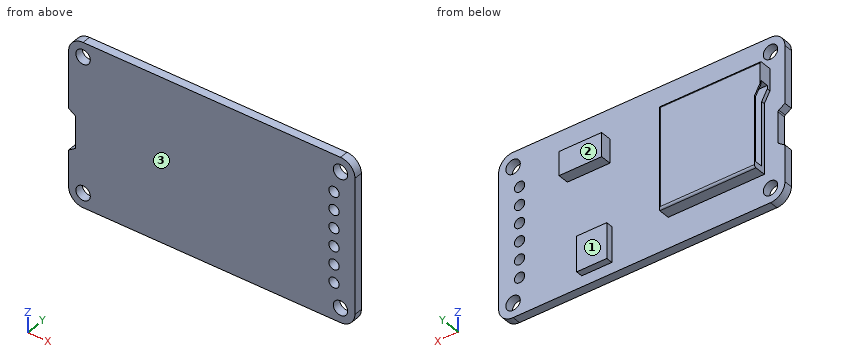
from build123d import *

# Parameters (mm, degrees)
ESQUISSE1_R                         = 1.05
PLAQUE_DEPTH                        = 1.24
CARTE_SD_DEPTH                      = 1.91
ESQUISSE4_W                         = 6.2
ESQUISSE4_H                         = 3.48
PUCE_DEPTH                          = 1.6
ESQUISSE7_W                         = 4.38
ESQUISSE7_H                         = 5.16
PUCE_2_DEPTH                        = 0.98
ESQUISSE8_R                         = 0.75
ENL_V_MAT_EXTRU_1_DEPTH             = 25.084021674
ESQUISSE9_W                         = 11.3
ESQUISSE9_H                         = 1.2
ENL_V_MAT_EXTRU_3_DEPTH             = 11.8
ENL_V_MAT_EXTRU_3_DIRECTION_2_REACH = 42.597
CONG_1_R                            = 0.3


with BuildPart() as part:
    # Esquisse1 → Plaque (new body)
    with BuildSketch(Plane(origin=(0, 0, 0), x_dir=(1, 0, 0), z_dir=(0, 1, 0))):
        with BuildLine():
            Line((-18.74, 11.92), (18.74, 11.92))
            ThreePointArc((18.74, 11.92), (20.22492424, 11.30492424), (20.84, 9.82))
            Line((20.84, 9.82), (20.84, -9.82))
            ThreePointArc((20.84, -9.82), (20.22492424, -11.30492424), (18.74, -11.92))
            Line((18.74, -11.92), (-18.74, -11.92))
            ThreePointArc((-18.74, -11.92), (-20.22492424, -11.30492424), (-20.84, -9.82))
            Line((-20.84, -9.82), (-20.84, -1.48))
            Line((-20.84, -1.48), (-19.951399946, -0.888062551))
            ThreePointArc((-19.951399946, -0.888062551), (-19.869602616, -0.798004209), (-19.84, -0.68))
            Line((-19.84, -0.68), (-19.84, 3.72))
            ThreePointArc((-19.84, 3.72), (-19.869602616, 3.838004209), (-19.951399946, 3.928062551))
            Line((-19.951399946, 3.928062551), (-20.84, 4.52))
            Line((-20.84, 4.52), (-20.84, 9.82))
            ThreePointArc((-20.84, 9.82), (-20.22492424, 11.30492424), (-18.74, 11.92))
        make_face()
        with Locations(Location((-18.74, 9.82, 0), (0, 0, 270))):
            Circle(ESQUISSE1_R, mode=Mode.SUBTRACT)
        with Locations(Location((18.74, 9.82, 0), (0, 0, 270))):
            Circle(ESQUISSE1_R, mode=Mode.SUBTRACT)
        with Locations(Location((-18.74, -9.82, 0), (0, 0, 270))):
            Circle(ESQUISSE1_R, mode=Mode.SUBTRACT)
        with Locations(Location((18.74, -9.82, 0), (0, 0, 270))):
            Circle(ESQUISSE1_R, mode=Mode.SUBTRACT)
    extrude(amount=PLAQUE_DEPTH)

    # Esquisse2 → Carte SD (add)
    with BuildSketch(Plane(origin=(0, 1.24, 0), x_dir=(1, 0, 0), z_dir=(0, 1, 0))):
        Polygon((-18.66, -7.44), (-3.84, -7.44), (-3.84, 7.44), (-17.84, 7.44), (-17.84, -2.756314418), (-18.66, -4.24), align=None)
    extrude(amount=CARTE_SD_DEPTH)

    # Esquisse4 → Puce (add)
    with BuildSketch(Plane(origin=(0, 1.24, 0), x_dir=(1, 0, 0), z_dir=(0, 1, 0))):
        with Locations((7.74, -5.86)):
            Rectangle(ESQUISSE4_W, ESQUISSE4_H)
    extrude(amount=PUCE_DEPTH)

    # Esquisse7 → Puce 2 (add)
    with BuildSketch(Plane(origin=(0, 1.24, 0), x_dir=(1, 0, 0), z_dir=(0, 1, 0))):
        with Locations((6.55, 7.74)):
            Rectangle(ESQUISSE7_W, ESQUISSE7_H)
    extrude(amount=PUCE_2_DEPTH)

    # Esquisse8 → Enlèv. mat.-Extru.1 (cut, through all)
    with BuildSketch(Plane(origin=(0, 1.24, 0), x_dir=(1, 0, 0), z_dir=(0, 1, 0))):
        with Locations(Location((17.79, 6.57, 0), (0, 0, 270))):
            Circle(ESQUISSE8_R)
        with Locations(Location((17.79, 3.95, 0), (0, 0, 270))):
            Circle(ESQUISSE8_R)
        with Locations(Location((17.79, 1.33, 0), (0, 0, 270))):
            Circle(ESQUISSE8_R)
        with Locations(Location((17.79, -1.29, 0), (0, 0, 270))):
            Circle(ESQUISSE8_R)
        with Locations(Location((17.79, -3.91, 0), (0, 0, 270))):
            Circle(ESQUISSE8_R)
        with Locations(Location((17.79, -6.53, 0), (0, 0, 270))):
            Circle(ESQUISSE8_R)
    extrude(amount=-ENL_V_MAT_EXTRU_1_DEPTH, mode=Mode.SUBTRACT)

    # Esquisse9 → Enlèv. mat.-Extru.3 (cut)
    with BuildSketch(Plane.ZY.offset(17.84)):
        with Locations((-0.92, 2.35)):
            Rectangle(ESQUISSE9_W, ESQUISSE9_H)
    extrude(amount=-ENL_V_MAT_EXTRU_3_DEPTH, mode=Mode.SUBTRACT)

    # Enlèv. mat.-Extru.3 direction 2: up to this face of the body (flat: up to its plane)
    enl_v_mat_extru_3_direction_2_end = Plane(part.part.faces().sort_by_distance((-18.66, 2.195, 5.84))[0])
    # Esquisse9 → Enlèv. mat.-Extru.3 direction 2 (cut, up to the picked face)
    with BuildSketch(Plane.ZY.offset(17.84), mode=Mode.PRIVATE) as enl_v_mat_extru_3_direction_2_sk1:
        with Locations((-0.92, 2.35)):
            Rectangle(ESQUISSE9_W, ESQUISSE9_H)
    enl_v_mat_extru_3_direction_2_tool1 = split(extrude(enl_v_mat_extru_3_direction_2_sk1.sketch, amount=ENL_V_MAT_EXTRU_3_DIRECTION_2_REACH, mode=Mode.PRIVATE), bisect_by=enl_v_mat_extru_3_direction_2_end, keep=Keep.BOTH, mode=Mode.PRIVATE)
    add(enl_v_mat_extru_3_direction_2_tool1.solids().sort_by(Axis((-17.84, 2.35, -0.92), (-1, 0, 0)))[0], mode=Mode.SUBTRACT)

    # Congé1
    cong_1_edges = [part.edges().sort_by_distance(p)[0] for p in [
        (-11.25, 3.15, 7.44),
        (-3.84, 3.15, 0),
        (-10.84, 3.15, -7.44),
    ]]
    fillet(cong_1_edges, radius=CONG_1_R)


solid = part.part
The listing builds one solid part. Answer for the finished solid, in the listing's coordinates (mm). Face numbers are marked on the shaded views. A direction names the side the tool comes from. Give positions to 0.01 mm unless a question says otherwise; leave off trailing zeros. Loops run counter-clockwise (first coordinate to the right, second up) from the corner with the lowest first, then second, coordinate; pieces in that order, holes last. Notation, with made-up numbers: (-26, -21) - (-20, -21) arc R20 cw to (-20, 4) - close; hole circle Ø6 at (31.5, 52). An arc over 180 degrees is marked (long way). Answer as a JSON object with one key per item and string values.
1. A cutting plane is placed at C-C (z = -9.25). Write down the section's boundary in (x, y), then the cut area to 3 significant figures.
Determined:
{"outline": "(-20.84, 0) - (-19.62, 0) - (-19.62, 1.24) - (-20.84, 1.24) - close; (-17.86, 0) - (17.86, 0) - (17.86, 1.24) - (8.74, 1.24) - (8.74, 2.22) - (4.36, 2.22) - (4.36, 1.24) - (-17.86, 1.24) - close; (19.62, 0) - (20.84, 0) - (20.84, 1.24) - (19.62, 1.24) - close", "area": "51.6 mm²"}
2. Flat-ended cylindrical pins translate along their axes: pin 1 Ø12 at (x, z) = (9, -1.5) entering from +Y; pin 2 Ø1.3 at (y, z) = (2.5, 5) entering from -X; pin 3 Ø1.3 at (x, y) = (-12.5, 2) entering from -Z. Find the tip coordinate at first contact, or state that the pin passes through.
Determined:
{"pin 1": "y = 2.84", "pin 2": "x = -18.66", "pin 3": "z = -7.44"}
3. A cutting plane is placed at B-B (x = -11). Write down the section's boundary in (y, z), then the cut area to 3 significant figures.
Determined:
{"outline": "(0, -11.92) - (1.24, -11.92) - (1.24, -7.44) - (2.85, -7.44) arc R0.3 ccw to (3.15, -7.14) - (3.15, 7.14) arc R0.3 ccw to (2.85, 7.44) - (1.24, 7.44) - (1.24, 11.92) - (0, 11.92) - close; hole (1.75, -6.57) - (2.95, -6.57) - (2.95, 4.73) - (1.75, 4.73) - close", "area": "44.4 mm²"}
4. A cutting plane is placed at A-A (z = 6.53). Write down the section's boundary in (x, y), then the cut area to 3 significant figures.
Determined:
{"outline": "(-20.84, 0) - (17.04, 0) - (17.04, 1.24) - (10.84, 1.24) - (10.84, 2.84) - (4.64, 2.84) - (4.64, 1.24) - (-3.84, 1.24) - (-3.84, 2.85) arc R0.3 ccw to (-4.14, 3.15) - (-18.66, 3.15) - (-18.66, 1.24) - (-20.84, 1.24) - close; (18.54, 0) - (20.84, 0) - (20.84, 1.24) - (18.54, 1.24) - close", "area": "88.0 mm²"}
5. A cutting plane is placed at D-D (x = 14.5). Write down the section's boundary in (y, z), then the cut area to 3 significant figures.
Determined:
{"outline": "(0, -11.92) - (1.24, -11.92) - (1.24, 11.92) - (0, 11.92) - close", "area": "29.6 mm²"}
6. For the marked faces 1, 2 and 3, determine the directions among +Z, -Z, +X, -X, +Y, -Y from which every point of the face is accessible in a straight line to the end or side of a thin tool.
Determined:
{"face 1": "-Z, +X, +Y", "face 2": "+Z, -Z, +X, +Y", "face 3": "+Z, -Z, +X, -X, -Y"}
7. Find the intervals of material crossed by L1, parallel to X at y = 0.6, z = 9.82; L2, parallel to Z at x = 6.5, y = 2; L3, parallel to Y at x = 7, z = -7.25, in increasing order. Write a range as [from, to].
Determined:
{"L1": "[-20.84, -19.79], [-17.69, 17.69], [19.79, 20.84]", "L2": "[-10.32, -5.16], [4.12, 7.6]", "L3": "[0, 2.22]"}
